Here's how the part is built. I have some questions about the finished solid (model axes, mm). A direction names the side the tool comes from. Round coordinates to 2 decimals unless told otherwise and drop trailing zeros. Loops run counter-clockwise (first coordinate to the right, second up) from the corner with the lowest first, then second, coordinate; pieces in that order, holes last. Notation, with made-up numbers: M -5,19 L 49,19 A15 ccw 49,44 Z; hole C -13.5,25.25 d11. An arc over 180 degrees is marked long. Write each question's results on one line, items separated by ' | '. Start each with the question number.
```python
from build123d import *

# Parameters (mm, degrees)
CUT_EXTRUDE1_DEPTH      = 32.981303132
CUT_EXTRUDE1_DEPTH_BACK = 32.981303132
SKETCH4_W               = 44.770884432
SKETCH4_H               = 10.69042287
SKETCH6_W               = 30.665330586
SKETCH6_H               = 1
BOSS_EXTRUDE1_DEPTH     = 21.05
SKETCH8_W               = 44.013591964
SKETCH8_H               = 26.255140404
CUT_EXTRUDE2_DEPTH      = 1
SKETCH9_W               = 50.816359418
SKETCH9_H               = 30.548951937
CUT_EXTRUDE3_DEPTH      = 1
CUT_EXTRUDE4_REACH      = 35.955
SKETCH10_R              = 5


with BuildPart() as part:
    # Sketch3 → Revolve1 (revolve)
    with BuildSketch(Plane.XY):
        Polygon((-7.025, 18.366712654), (-8.025, 18.366712654), (-17.025, -2.683287346), (-16.025, -2.683287346), align=None)
    revolve(axis=Axis((0, 50, 0), (0, -1, 0)))

    # Sketch4 → Cut-Extrude1 (cut, two sides: drawn at the far end of the back side and taken through both)
    with BuildSketch(Plane(origin=(0, 18.366712654, 0), x_dir=(1, 0, 0), z_dir=(0, 1, 0)).offset(-CUT_EXTRUDE1_DEPTH_BACK)):
        with Locations((0.720276718, -12.745211435)):
            Rectangle(SKETCH4_W, SKETCH4_H)
    extrude(amount=CUT_EXTRUDE1_DEPTH + CUT_EXTRUDE1_DEPTH_BACK, mode=Mode.SUBTRACT)

    # Sketch6 → Boss-Extrude1 (add)
    with BuildSketch(Plane.XZ.offset(2.683287346)):
        with Locations((0, 6.9)):
            Rectangle(SKETCH6_W, SKETCH6_H)
    extrude(amount=-BOSS_EXTRUDE1_DEPTH)

    # Sketch7 → Cut-Revolve1 (revolve, cut)
    with BuildSketch(Plane(origin=(0, 0, 0), x_dir=(0, 0, -1), z_dir=(1, 0, 0))):
        Polygon((8.025, 18.366712654), (17.025, -2.683287346), (18.600289965, -2.683287346), (18.600289965, 18.366712654), align=None)
    revolve(axis=Axis((0, 14.930838331, 0), (0, -1, 0)), mode=Mode.SUBTRACT)

    # Sketch8 → Cut-Extrude2 (cut)
    with BuildSketch(Plane(origin=(0, 18.366712654, 0), x_dir=(1, 0, 0), z_dir=(0, 1, 0))):
        with Locations((-2.588663139, 4.329260992)):
            Rectangle(SKETCH8_W, SKETCH8_H)
    extrude(amount=-CUT_EXTRUDE2_DEPTH, mode=Mode.SUBTRACT)

    # Sketch9 → Cut-Extrude3 (cut)
    with BuildSketch(Plane.XZ.offset(2.683287346)):
        with Locations((0.819476292, -3.706436551)):
            Rectangle(SKETCH9_W, SKETCH9_H)
    extrude(amount=-CUT_EXTRUDE3_DEPTH, mode=Mode.SUBTRACT)

    # Sketch10 → Cut-Extrude4 (cut, up to next)
    with BuildSketch(Plane.XY.offset(7.4), mode=Mode.PRIVATE) as cut_extrude4_sk1:
        with Locations((0, 7.016712654)):
            Circle(SKETCH10_R)
    cut_extrude4_tool1 = extrude(cut_extrude4_sk1.sketch, amount=-CUT_EXTRUDE4_REACH, mode=Mode.PRIVATE) & part.part
    add(cut_extrude4_tool1.solids().sort_by_distance((0, 7.016713, 7.4))[0], mode=Mode.SUBTRACT)


solid = part.part
```
1. I want a section at A-A on z = 0. List the corners of the cut face in (x, y) for me.
2. Which directions (+Z, -Z, +X, -X, +Y, -Y) give clear straight access to the entire face, cutting with the end or side of a thin tool? Please do faces 1 (the face through (0, 1, 6.4)), 2 (the face through (0, 1, 7.4)).
3. If we mould it in two halves opening along Z, with no side actions, what happens to faces 3 (the face through (-0.385, 10.092, -10.556)), 4 (the face through (-0.398, 11.942, -10.765)), 5 (the face through (2.69, 11.23, 6.91))? For each: released by +Z, released by -Z, zero draft, split by the parting line, or undercut.
4. I want a section at B-B on x = 0. List the corners of the cut face in (y, z) for me, plus the area to 3 significant figures.
5. I need wall thicknesses on line 1 along Y through (x, z) = (0, 7); line 2 along X through (y, z) = (5, -4); line 3 along X through (y, z) = (13.5, 3.5). Which ranges of each line are inside material? Lowest first, please.
6. I want a section at D-D on y = 13.75. List the corners of the cut face in (x, z) for me, plus the area to 3 significant figures.
7. I want a section at C-C on y = 3. List the corners of the cut face in (x, z) for me.
8. For pin 1 (8 mm diameter, centred on y = 11, z = -6.5, fed in from +X); pin 2 (8 mm diameter, centred on x = 12, z = -9.5, fed in from +Y); pin 3 (3 mm diameter, centred on y = 7, z = -8.5, fed in from -X), each with a flat end and sliding along its axis, tell me the tip position at first contact or that it passes through.
Outcome:
1) outline: M -16.6,-1.68 L -15.6,-1.68 L -7.45,17.37 L -8.45,17.37 Z; M 7.45,17.37 L 15.6,-1.68 L 16.6,-1.68 L 8.45,17.37 Z
2) face 1: -Y | face 2: +Z, +X, -X, +Y, -Y
3) face 3: undercut | face 4: split by the parting line | face 5: zero draft
4) outline: M -1.68,-16.6 L 17.37,-8.45 L 17.37,-7.45 L -1.68,-15.6 Z; M -1.68,6.4 L 2.02,6.4 L 2.02,7.4 L -1.68,7.4 Z; M 12.02,6.4 L 17.37,6.4 L 17.37,7.4 L 12.02,7.4 Z | area: 28.1 mm2
5) line 1: -1.68 to 2.02, 12.02 to 17.37 | line 2: -13.14 to -12.1, 12.1 to 13.14 | line 3: -9.48 to -8.41, 8.41 to 9.48
6) outline: M -6.72,7.4 A10 ccw long 6.72,7.4 Z; hole M -6.33,6.4 A9 ccw long 6.33,6.4 Z | area: 58.3 mm2
7) outline: M -12.58,7.4 A14.6 ccw long 12.58,7.4 L 2.98,7.4 L 2.98,6.4 L 11.99,6.4 A13.6 cw long -11.99,6.4 L -2.98,6.4 L -2.98,7.4 Z
8) pin 1: x = 11.85 | pin 2: y = 10.69 | pin 3: x = -11.08
